Part model, mm, in its own coordinate system. Face numbers are marked on the shaded views. A direction names the side the tool comes from. Coordinates: 2 decimals unless noted, no trailing zeros. Order: outer loops, then holes, each group sorted by start corner. A loop starts at its lowest first (then second) coordinate and runs counter-clockwise, first axis right, second up. Notation, with made-up numbers: (-14.5, -37.5) - (31.5, -37.5) arc R33 cw to (31.5, -1.5) - close; hole circle Ø1 at (45, -17.75). An arc over 180 degrees is marked (long way). Use a Markdown table: item, result. Add a question column.
1) Wall check: L1, parallel to Y at x = 0, z = 1.65 (3 decimals); L2, parallel to Y at x = 0, z = -10 (3 decimals); L3, parallel to Y at x = 0, z = 4 (3 decimals). Give the ranges that are in metal, low to high. Write a range as [from, to].
2) Saw through at D-D on z = -36.5. List the corners of the cut face in (x, y), then the cut area to 3 significant figures.
3) Two-plate mould, pull along X, no slides. Class the marked faces 1, 2 and 3: +X half, -X half, draft (parallel to the pull), parting line (faces both ways), or undercut.
4) Saw through at A-A on z = -19. List the corners of the cut face in (x, y) (3 decimals), then the cut area to 3 significant figures.
5) Saw through at C-C on y = 39.5. List the corners of the cut face in (x, z).
6) Tool access for the marked faces 4 and 5: list every direction of +Z, -Z, +X, -X, +Y, -Y with a clear straight run to the whole face (end or side of a thin tool).
7) Saw through at B-B on x = 32. List the corners of the cut face in (y, z).
8) Drop flat-ended pins along their axis: P1, Ø14.5, axis at x = -0.5, y = 10.5, coming from the +Z side; P2, Ø3, axis at x = -12.5, y = -19.5, coming from the -Z side; P3, Ø0.6, axis at x = 23.5, y = -1, coming from the -Z side; P4, Ø5, axis at y = 8, z = -14, coming from the -X side. Give the stop position or say it passes through.
```python
from build123d import *
from build123d.topology import SkipClean

# Parameters (mm, degrees)
SKETCH1_R                = 23.975
BOSS_EXTRUDE1_DEPTH      = 5
BOSS_EXTRUDE6_DEPTH      = 45
CUT_EXTRUDE3_DEPTH       = 42
BOSS_EXTRUDE3_DEPTH      = 10
CUT_EXTRUDE2_DEPTH       = 94.005376189
CIRPATTERN1_COUNT        = 3
SKETCH3_R                = 22.25
CUT_EXTRUDE1_DEPTH       = 94.005376189
BOSS_EXTRUDE4_START      = -0.2
SKETCH5_R                = 23.975
SKETCH5_R_2              = 20
BOSS_EXTRUDE4_DEPTH      = 0.2
SKETCH6_R                = 20.8
SKETCH6_R_2              = 20
BOSS_EXTRUDE5_DEPTH      = 1.7
SKETCH8_W                = 34
SKETCH8_H                = 2.5
M3_START                 = -55
M3_CLEARANCE_SLOT3_DEPTH = 4
SKETCH14_R               = 5
CUT_EXTRUDE4_DEPTH       = 97.306801421
FILLET3_R                = 2
CHAMFER1_SIZE            = 0.8


# Read off the part's stored shape, not the designer's step: M3 Clearance Slot3
with BuildPart() as part:
    # Sketch1 → Boss-Extrude1 (new body)
    with BuildSketch(Plane.XY):
        Polygon((-45, -45), (-45, -55), (45, -55), (45, -45), (45, 45), (-45, 45), align=None)
        Circle(SKETCH1_R, mode=Mode.SUBTRACT)
    extrude(amount=BOSS_EXTRUDE1_DEPTH)

    # Sketch9 → Boss-Extrude6 (add, symmetric)
    with BuildSketch(Plane(origin=(0, 0, 0), x_dir=(0, 0, -1), z_dir=(1, 0, 0))):
        with BuildLine():
            Line((0, 45), (0, -55))
            Line((0, -55), (60, -55))
            Line((60, -55), (60, -48))
            ThreePointArc((60, -48), (58.535533906, -44.464466094), (55, -43))
            Line((55, -43), (29.730670818, -43))
            ThreePointArc((29.730670818, -43), (20.024502844, -39.436358829), (14.930241511, -30.438707102))
            Line((14.930241511, -30.438707102), (2.844959748, 42.906451184))
            ThreePointArc((2.844959748, 42.906451184), (1.995916193, 44.406059805), (0.37822153, 45))
            Line((0.37822153, 45), (0, 45))
        make_face()
    extrude(amount=BOSS_EXTRUDE6_DEPTH, both=True)

    # Sketch10 → Cut-Extrude3 (cut, symmetric)
    with BuildSketch(Plane(origin=(0, 0, 0), x_dir=(0, 0, -1), z_dir=(1, 0, 0))):
        Polygon((0, 45), (0, -51), (62.788214541, -51), (2.5, 45), align=None)
    extrude(amount=CUT_EXTRUDE3_DEPTH, both=True, mode=Mode.SUBTRACT)

    # Sketch2 → Boss-Extrude3 (add)
    with BuildSketch(Plane.ZY.offset(-23.975)):
        Polygon((0, -2.4), (3.3, -2.4), (3.3, 14.5), (2.5, 14.5), (1.8, 0), (0, 0), align=None)
    boss_extrude3 = extrude(amount=BOSS_EXTRUDE3_DEPTH)

    # Sketch4 → Cut-Extrude2 (cut, through all)
    with BuildSketch(Plane.XY):
        with BuildLine():
            Line((16.63749335, 17.262515461), (0, 0))
            Line((0, 0), (19.359883897, 14.141977248))
            ThreePointArc((19.359883897, 14.141977248), (18.066190297, 15.761135529), (16.63749335, 17.262515461))
        make_face()
    cut_extrude2 = extrude(amount=CUT_EXTRUDE2_DEPTH, mode=Mode.SUBTRACT)

    # CirPattern1: Boss-Extrude3, Cut-Extrude2 ×3 about axis
    cirpattern1_axis = Axis((0, 0, 0), (0, 0, 1))
    add([boss_extrude3.rotate(cirpattern1_axis, i * 360 / CIRPATTERN1_COUNT) for i in range(1, CIRPATTERN1_COUNT)])
    add([cut_extrude2.rotate(cirpattern1_axis, i * 360 / CIRPATTERN1_COUNT) for i in range(1, CIRPATTERN1_COUNT)], mode=Mode.SUBTRACT)

    # Sketch3 → Cut-Extrude1 (cut, through all)
    with BuildSketch(Plane.XY):
        Circle(SKETCH3_R)
    extrude(amount=CUT_EXTRUDE1_DEPTH, mode=Mode.SUBTRACT)

    # Sketch5 → Boss-Extrude4 (add)
    with BuildSketch(Plane.XY.offset(3.3).offset(BOSS_EXTRUDE4_START)):
        with Locations(Location((0, 0, 0), (0, 0, 180))):
            Circle(SKETCH5_R)
        Circle(SKETCH5_R_2, mode=Mode.SUBTRACT)
    extrude(amount=BOSS_EXTRUDE4_DEPTH)

    # Sketch6 → Boss-Extrude5 (add)
    with BuildSketch(Plane.XY.offset(3.3)):
        with Locations(Location((0, 0, 0), (0, 0, 180))):
            Circle(SKETCH6_R)
        Circle(SKETCH6_R_2, mode=Mode.SUBTRACT)
    extrude(amount=BOSS_EXTRUDE5_DEPTH)

    # Sketch8 → Revolve1 (revolve)
    with SkipClean():  # the faces are left unmerged after this step: merging them gives an invalid solid
        with BuildSketch(Plane(origin=(0, 0, 0), x_dir=(0, 0, -1), z_dir=(1, 0, 0)), mode=Mode.PRIVATE) as revolve1_sk:
            with Locations((17, 25.225)):
                Rectangle(SKETCH8_W, SKETCH8_H)
        revolve(revolve1_sk.sketch.rotate(Axis((0, 0, 0), (0, 0, 1)), 90), axis=Axis((0, 0, 0), (0, 0, 1)))

    # M3 Clearance Slot3 outline → M3 Clearance Slot3 (cut)
    with SkipClean():  # the faces are left unmerged after this step: merging them gives an invalid solid
        with BuildSketch(Plane(origin=(0, 0, 0), x_dir=(1, 0, 0), z_dir=(0, 1, 0)).offset(M3_START)):
            with BuildLine():
                Line((33.7, 41.7), (33.7, 53.122760777))
                ThreePointArc((33.7, 53.122760777), (32, 54.822760777), (30.3, 53.122760777))
                Line((30.3, 53.122760777), (30.3, 41.7))
                ThreePointArc((30.3, 41.7), (32, 40), (33.7, 41.7))
            make_face()
            with BuildLine():
                Line((-30.3, 41.7), (-30.3, 53.122760777))
                ThreePointArc((-30.3, 53.122760777), (-32, 54.822760777), (-33.7, 53.122760777))
                Line((-33.7, 53.122760777), (-33.7, 41.7))
                ThreePointArc((-33.7, 41.7), (-32, 40), (-30.3, 41.7))
            make_face()
        extrude(amount=M3_CLEARANCE_SLOT3_DEPTH, mode=Mode.SUBTRACT)

    # Sketch14 → Cut-Extrude4 (cut, through all)
    with SkipClean():  # the faces are left unmerged after this step: merging them gives an invalid solid
        with BuildSketch(Plane.XY.offset(5)):
            with Locations((0, -43)):
                Circle(SKETCH14_R)
        extrude(amount=-CUT_EXTRUDE4_DEPTH, mode=Mode.SUBTRACT)

    # Fillet3
    fillet3_edges = [part.edges().sort_by_distance(p)[0] for p in [
        (42, -3, 0),
        (0, -51, 0),
        (-42, -3, 0),
        (42, -51, -30),
        (-42, -51, -30),
    ]]
    fillet(fillet3_edges, radius=FILLET3_R)

    # Chamfer1
    chamfer1_edges = [part.edges().sort_by_distance(p)[0] for p in [
        (45, -55, -27.5),
        (-45, -55, -27.5),
        (0, -55, 5),
        (0, -55, -60),
        (32, -55, -54.822760777),
        (32, -55, -40),
        (30.3, -55, -47.411380389),
        (33.7, -55, -47.411380389),
        (-33.7, -55, -47.411380389),
        (-32, -55, -54.822760777),
        (-32, -55, -40),
        (-30.3, -55, -47.411380389),
    ]]
    chamfer(chamfer1_edges, length=CHAMFER1_SIZE)


solid = part.part
```
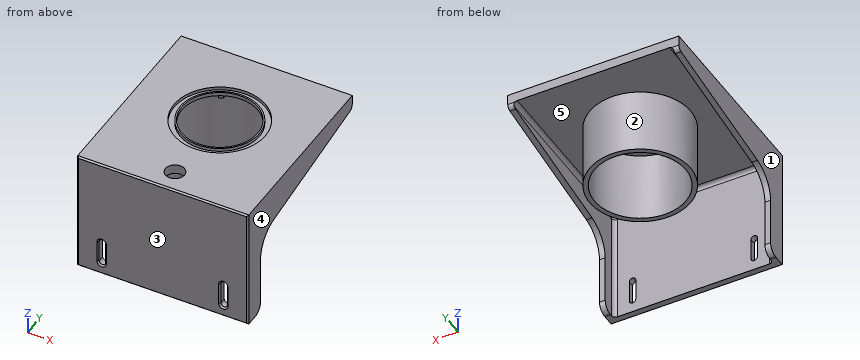
Results are:
| question | item | result |
|---|---|---|
| 1 | L1 | [-55, -48], [-38, -23.975], [23.975, 45] |
| 1 | L2 | [-55, -51], [-26.475, -23.975], [23.975, 26.475] |
| 1 | L3 | [-55, -48], [-38, -23.975], [-20.8, -20], [20, 20.8], [23.975, 45] |
| 2 | outline | (-45, -54.2) - (-44.2, -55) - (44.2, -55) - (45, -54.2) - (45, -43) - (42, -43) - (42, -49) arc R2 cw to (40, -51) - (-40, -51) arc R2 cw to (-42, -49) - (-42, -43) - (-45, -43) - close |
| 2 | area | 409 mm2 |
| 3 | face 1 | -X half |
| 3 | face 2 | undercut |
| 3 | face 3 | draft |
| 4 | outline | (-45, -54.2) - (-44.2, -55) - (44.2, -55) - (45, -54.2) - (45, -38.481) - (42, -38.481) - (42, -49) arc R2 cw to (40, -51) - (-40, -51) arc R2 cw to (-42, -49) - (-42, -38.481) - (-45, -38.481) - close; circle Ø52.95 at (0, 0); hole circle Ø47.95 at (0, 0) |
| 4 | area | 832 mm2 |
| 5 | outline | (-45, -3.41) - (-42, -3.41) - (-42, -2) arc R2 cw to (-40, 0) - (40, 0) arc R2 cw to (42, -2) - (42, -3.41) - (45, -3.41) - (45, 5) - (-45, 5) - close |
| 6 | face 4 | +Z, -Z, +X, +Y, -Y |
| 6 | face 5 | -Z |
| 7 | outline | (-55, -59.2) - (-54.2, -60) - (-51, -60) - (-51, -54.82) - (-54.2, -54.82) - (-55, -55.62) - close; (-55, -39.2) - (-54.2, -40) - (-51, -40) - (-51, -2) arc R2 cw to (-49, 0) - (45, 0) - (45, 5) - (-54.2, 5) - (-55, 4.2) - close |
| 8 | P1 | through |
| 8 | P2 | z = -34 |
| 8 | P3 | z = 0 |
| 8 | P4 | x = -25.9 |
